Read the model definition and answer for the solid it produces. Units are mm, in the model's axes. Face numbers are marked on the shaded views. A direction names the side the tool comes from. Coordinates: 2 decimals unless noted, no trailing zeros. Order: outer loops, then holes, each group sorted by start corner. A loop starts at its lowest first (then second) coordinate and runs counter-clockwise, first axis right, second up. Notation, with made-up numbers: (62.25, 48.5) - (103.25, 48.5) arc R24 cw to (103.25, 83.5) - close; hole circle Ø10 at (7.5, -27.75). An arc over 180 degrees is marked (long way). Write item = value, one per line.
from build123d import *

# Parameters (mm, degrees)
F0_R     = 3.81
F1_DEPTH = 15.24


with BuildPart() as f1:
    # F0 (on Top) → F1 (new body)
    with BuildSketch(Plane.XY):
        with BuildLine():
            ThreePointArc((0, 5.08), (1.487898, 1.487898), (5.08, 0))
            Line((5.08, 0), (28.9306, 0))
            ThreePointArc((28.9306, 0), (32.522702, 1.487898), (34.0106, 5.08))
            Line((34.0106, 5.08), (34.0106, 109.22))
            ThreePointArc((34.0106, 109.22), (32.522702, 112.812102), (28.9306, 114.3))
            Line((28.9306, 114.3), (5.08, 114.3))
            ThreePointArc((5.08, 114.3), (1.487898, 112.812102), (0, 109.22))
            Line((0, 109.22), (0, 5.08))
        make_face()
        with Locations((25.1206, 11.2776)):
            Circle(F0_R, mode=Mode.SUBTRACT)
        with Locations((8.89, 103.0224)):
            Circle(F0_R, mode=Mode.SUBTRACT)
        with BuildLine():
            ThreePointArc((17.0053, 104.14), (18.493198, 107.732102), (22.0853, 109.22))
            Line((22.0853, 109.22), (24.6253, 109.22))
            ThreePointArc((24.6253, 109.22), (28.217402, 107.732102), (29.7053, 104.14))
            Line((29.7053, 104.14), (29.7053, 88.9))
            ThreePointArc((29.7053, 88.9), (28.217402, 85.307898), (24.6253, 83.82))
            Line((24.6253, 83.82), (22.0853, 83.82))
            ThreePointArc((22.0853, 83.82), (18.493198, 85.307898), (17.0053, 88.9))
            Line((17.0053, 88.9), (17.0053, 104.14))
        make_face(mode=Mode.SUBTRACT)
    extrude(amount=F1_DEPTH)


solid = f1.part
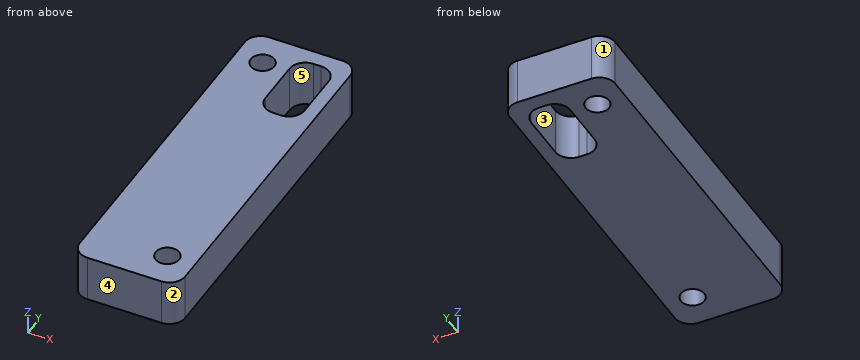
1) The part is cut by section B-B (y = 95). Determine the outline of the cut face in (x, z).
Returned:
outline = (0, 0) - (17.01, 0) - (17.01, 15.24) - (0, 15.24) - close; (29.71, 0) - (34.01, 0) - (34.01, 15.24) - (29.71, 15.24) - close
2) The part is cut by section C-C (z = 8). Determine the outline of the cut face in (x, y).
Returned:
outline = (0, 5.08) arc R5.08 ccw to (5.08, 0) - (28.93, 0) arc R5.08 ccw to (34.01, 5.08) - (34.01, 109.22) arc R5.08 ccw to (28.93, 114.3) - (5.08, 114.3) arc R5.08 ccw to (0, 109.22) - close; hole circle Ø7.62 at (8.89, 103.02); hole (17.01, 88.9) arc R5.08 ccw to (22.09, 83.82) - (24.63, 83.82) arc R5.08 ccw to (29.71, 88.9) - (29.71, 104.14) arc R5.08 ccw to (24.63, 109.22) - (22.09, 109.22) arc R5.08 ccw to (17.01, 104.14) - close; hole circle Ø7.62 at (25.12, 11.28)
3) The part is cut by section A-A (x = 8.89). Determine the outline of the cut face in (y, z).
Returned:
outline = (0, 0) - (99.21, 0) - (99.21, 15.24) - (0, 15.24) - close; (106.83, 0) - (114.3, 0) - (114.3, 15.24) - (106.83, 15.24) - close
4) Straight lines are drawn through the part: line 1 along Y through (x, z) = (9, 4.5); line 2 along X through (y, z) = (99, 3); line 3 along Y through (x, z) = (10, 6.75). For each, find the intervals that lie inside material, in ascending order. Write a range as from..to.
Returned:
line_1 = 0..99.21, 106.83..114.3
line_2 = 0..17.01, 29.71..34.01
line_3 = 0..99.38, 106.67..114.3
5) Determine the mould class of the marked faces 1, 2 and 3 for opening direction X: pulls with the +X half, pulls with the -X half, needs draft (parallel to the pull), parting line crosses it, or undercut.
Returned:
face_1 = pulls with the -X half
face_2 = pulls with the +X half
face_3 = undercut
6) For the marked faces 4 and 5, determine the directions among +Z, -Z, +X, -X, +Y, -Y from which every point of the face is accessible in a straight line to the end or side of a thin tool.
Returned:
face_4 = +Z, -Z, +X, -X, -Y
face_5 = +Z, -Z
